Autodesk Inventor part; units mm, degrees
ref_plane "YZ Plane" through (0, 0, 0) normal (1, 0, 0) x (0, 1, 0)
ref_plane "XZ Plane" through (0, 0, 0) normal (0, 1, 0) x (-1, 0, 0)
ref_plane "XY Plane" through (0, 0, 0) normal (0, 0, 1) x (1, 0, 0)
sketch "Base" plane through (0, 0, 0) normal (0, 0, 1) x (1, 0, 0)
  line L0 (0, 0) -> (0, -18) construction
  line L1 (0, -18) -> (2, -18)
  line L2 (2, -18) -> (4, -14.9841)
  line L3 (5, -3.4641) -> (3, 0)
  line L4 (3, 0) -> (0, 0)
  line L5 (4, -14.9841) -> (5, -3.4641)
  line L6 (0, -18) -> (0.8747, -13.5)
  line L7 (0.8747, -13.5) -> (0, 0)
  dimension "d0" = 18
  dimension "d1" = 3
  dimension "d2" = 2
  dimension "d3" = 5
  dimension "d8" = 4
  dimension "d12" = 120
  dimension "d14" = 11.52
  dimension "d23" = 13.5
  dimension "d24" = 79
extrude "BaseFeature" add sketch "Base" along normal blind 14
sketch "TopProfile" plane through (0.8747, -13.5, 0) normal (-0.9979, -0.0647, 0) x (0, 0, 1)
  line L0 (0, 9.7482) -> (14, 9.7482)
  line L1 (3, 13.5283) -> (11, 13.5283)
  line L2 (11, 13.5283) -> (14, 9.7482)
  line L3 (14, 9.7482) -> (10, -4.5633)
  line L4 (10, -4.5633) -> (4, -4.5633)
  line L5 (4, -4.5633) -> (0, 9.7482)
  line L6 (0, 9.7482) -> (3, 13.5283)
  line L7 (0, 13.5283) -> (14, 13.5283)
  line L8 (0, -4.5633) -> (14, -4.5633)
  point P0 (7, 13.5283)
  point P1 (7, -4.5633)
  dimension "d27" = 8
  dimension "d28" = 6
extrude "TopProfileFeature" cut sketch "TopProfile" along normal through all both and the other way through all keep common part
equation "\"d14\" = 0.64 * d0"
equation "\"d23\" = 0.75 * d0"
properties part number "DistalPhalangeIndexMiddle"
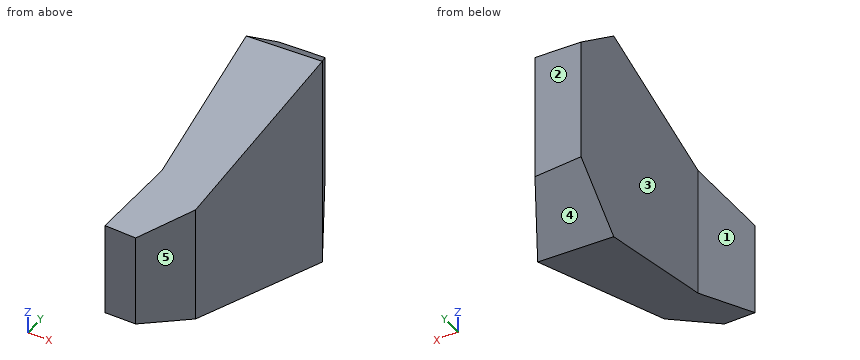
Geometry check sheet. Reference: the model listing, model coordinates, mm. Face numbers are marked on the shaded views. A direction names the side the tool comes from. Give positions to 0.01 mm unless a question says otherwise; leave off trailing zeros. Write each loop counter-clockwise with the first axis right and the second up, starting at its lowest first coordinate (ties: lowest second). Pieces come first, ordered by that corner, then holes.
1) Section check D-D, the plane x = 3.35. Record the boundary of the cut face in (y, z), and give its area (3 significant figures).
2) Section check C-C, the plane y = -9. Record the boundary of the cut face in (x, z), and give its area (3 significant figures).
3) Material ranges on L1, parallel to X at y = -13.25, z = 11.25; L2, parallel to Z at x = 1, y = -6.5; L3, parallel to Z at x = 1.35, y = -11, recorded low to high.
4) Release check for a two-part mould opening along Y. For the marked faces 3, 4 and 5 record: pulls with the +Y half, pulls with the -Y half, needs draft (parallel to the pull), parting line crosses it, or undercut.
5) Gauge pin test, flat ends, axial feed: pin 1 (1.5 mm diameter, centred on y = -11.5, z = 3.5, fed in from -X); pin 2 (1.5 mm diameter, centred on y = -11.5, z = 10.5, fed in from +X); pin 3 (3 mm diameter, centred on x = 1, y = -8.5, fed in from +Z). Record the tip position at first contact, or that the pin passes through.
6) Access from +Z, -Z, +X, -X, +Y, -Y to the whole of each face (thin tool, end or side, straight path). Record for the marked faces 1 and 2.
7) Section check B-B, the plane x = 0.55. Record the boundary of the cut face in (y, z), and give its area (3 significant figures).
Computed:
1. outline: (-15.96, 3.46) - (-3.57, 0) - (-0.61, 2.35) - (-0.61, 11.65) - (-3.57, 14) - (-15.96, 10.54) - close
1. area: 165 mm2
2. outline: (0.58, 1.46) - (4.52, 1.54) - (4.52, 12.46) - (0.58, 12.54) - close
2. area: 43.3 mm2
3. L1: x = 0.86 to 4.15
3. L2: z = 0.77 to 13.23
3. L3: z = 2.04 to 11.96
4. face 3: undercut
4. face 4: pulls with the +Y half
4. face 5: pulls with the -Y half
5. pin 1: stops at x = 0.7
5. pin 2: stops at x = 4.37
5. pin 3: stops at z = 13.09
6. face 1: +Z, -Z, -X
6. face 2: +Z, -Z, +X, -X, +Y
7. outline: (-18, 3.97) - (-15.17, 3.18) - (-15.17, 10.82) - (-18, 10.03) - close; (-8.49, 1.32) - (-3.75, 0) - (0, 2.97) - (0, 11.03) - (-3.75, 14) - (-8.49, 12.68) - close
7. area: 121 mm2
